from build123d import *

# Parameters (mm, degrees)
SKETCH_1_W          = 120
SKETCH_1_H          = 10
EXTRUDE_1_DEPTH     = 2
SKETCH_2_W          = 3
SKETCH_2_H          = 10
EXTRUDE_2_DEPTH     = 13
CUT_EXTRUDE_1_REACH = 119.073
SKETCH_3_R          = 1.575


with BuildPart() as part:
    # 草图1 → 凸台-拉伸1 (new body)
    with BuildSketch(Plane.XY):
        Rectangle(SKETCH_1_W, SKETCH_1_H)
    extrude(amount=EXTRUDE_1_DEPTH)

    # 草图2 → 凸台-拉伸2 (add)
    with BuildSketch(Plane.XY.offset(2)):
        with Locations((-54.5, 0)):
            Rectangle(SKETCH_2_W, SKETCH_2_H)
        with Locations((54.5, 0)):
            Rectangle(SKETCH_2_W, SKETCH_2_H)
    extrude(amount=EXTRUDE_2_DEPTH)

    # 切除-拉伸1: up to this face of the body (flat: up to its plane)
    cut_extrude_1_end = Plane(part.part.faces().sort_by_distance((-56, 0, 8.5))[0])
    # 草图3 → 切除-拉伸1 (cut, up to the picked face)
    with BuildSketch(Plane(origin=(56, 0, 0), x_dir=(0, 0, -1), z_dir=(1, 0, 0)), mode=Mode.PRIVATE) as cut_extrude_1_sk1:
        with Locations(Location((-11.5, 0, 0), (0, 0, 90))):
            Circle(SKETCH_3_R)
    cut_extrude_1_tool1 = split(extrude(cut_extrude_1_sk1.sketch, amount=-CUT_EXTRUDE_1_REACH, mode=Mode.PRIVATE), bisect_by=cut_extrude_1_end, keep=Keep.BOTH, mode=Mode.PRIVATE)
    add(cut_extrude_1_tool1.solids().sort_by(Axis((56, 0, 11.5), (-1, 0, 0)))[0], mode=Mode.SUBTRACT)


solid = part.part
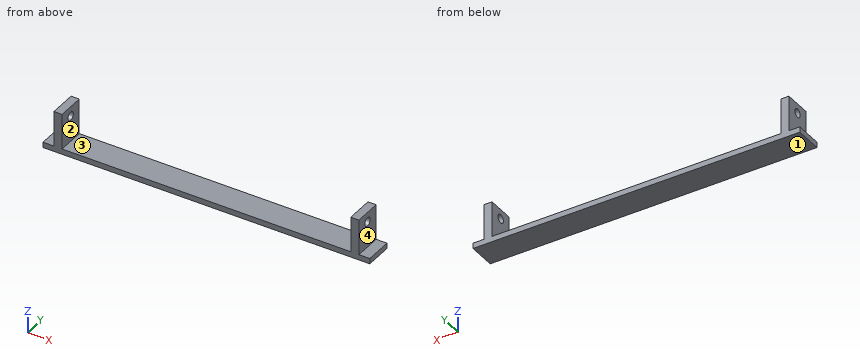
Work out the finished part from the listing and answer in its coordinate system (mm). Face numbers are marked on the shaded views. Give positions to 0.01 mm unless a question says otherwise; leave off trailing zeros. Loops run counter-clockwise (first coordinate to the right, second up) from the corner with the lowest first, then second, coordinate; pieces in that order, holes last. Notation, with made-up numbers: (-9, 23) - (14, 23) arc R27 ccw to (14, 53) - close; hole circle Ø1 at (8.5, -0.75). An arc over 180 degrees is marked (long way). Answer in a Markdown table with one row per item. Add a question column.
Q1. Consider line 1 along X through (y, z) = (-3.25, 11.25); line 2 along Z through (x, y) = (-55.25, 0) (3 decimals); line 3 along Z through (x, y) = (38, 2.75). Determine where each line is inside the solid, lowest interval first.
Q2. Each of these flat-tipped pins is pushed along its axis until it touches: P1, Ø3, axis at x = -7.5, y = 1.5, coming from the +Z side; P2, Ø5, axis at y = 1.5, z = 9.5, coming from the +X side; P3, Ø3, axis at y = 0.5, z = 6.5, coming from the -X side. Where does it stop, or does it pass through?
Q3. The part is cut by section B-B (z = 7.75). Determine the outline of the cut face in (x, y), and give its area (3 significant figures).
Q4. The part is cut by section C-C (x = 0.5). Determine the outline of the cut face in (y, z), and give its area (3 significant figures).
Q5. The part is cut by section A-A (y = 0). Determine the outline of the cut face in (x, z) (3 decimals), and give its area (3 significant figures).
Q6. Determine the mould class of the marked faces 1, 2, 3 and 4 for opening direction X: released by +X, released by -X, zero draft, split by the parting line, or undercut.
Solution:
| question | item | result |
|---|---|---|
| 1 | line 1 | x = -56 to -53, 53 to 56 |
| 1 | line 2 | z = 0 to 9.925, 13.075 to 15 |
| 1 | line 3 | z = 0 to 2 |
| 2 | P1 | stops at z = 2 |
| 2 | P2 | stops at x = 56 |
| 2 | P3 | stops at x = -56 |
| 3 | outline | (-56, -5) - (-53, -5) - (-53, 5) - (-56, 5) - close; (53, -5) - (56, -5) - (56, 5) - (53, 5) - close |
| 3 | area | 60.0 mm² |
| 4 | outline | (-5, 0) - (5, 0) - (5, 2) - (-5, 2) - close |
| 4 | area | 20.0 mm² |
| 5 | outline | (-60, 0) - (60, 0) - (60, 2) - (56, 2) - (56, 9.925) - (53, 9.925) - (53, 2) - (-53, 2) - (-53, 9.925) - (-56, 9.925) - (-56, 2) - (-60, 2) - close; (-56, 13.075) - (-53, 13.075) - (-53, 15) - (-56, 15) - close; (53, 13.075) - (56, 13.075) - (56, 15) - (53, 15) - close |
| 5 | area | 299 mm² |
| 6 | face 1 | zero draft |
| 6 | face 2 | undercut |
| 6 | face 3 | undercut |
| 6 | face 4 | released by +X |
